Here's how the part is built. I have some questions about the finished solid (model axes, mm). Face numbers are marked on the shaded views. A direction names the side the tool comes from. Give positions to 0.01 mm unless a question says otherwise; leave off trailing zeros. Write each loop counter-clockwise with the first axis right and the second up, starting at its lowest first coordinate (ties: lowest second). Pieces come first, ordered by that corner, then holes. Notation, with made-up numbers: (16.5, 16.5) - (60.5, 16.5) arc R27 cw to (60.5, 52.5) - close; hole circle Ø9 at (29.5, 27.25). An arc over 180 degrees is marked (long way). One line per item, written item: value. Start each with the question number.
1) Imagine slicing it at D-D on z = 35. Write out the boundary of the cut face in (x, y).
2) We'd pull the mould along Y, two halves only. Please class the marked faces 1, 2, 3 and 4: +Y half, -Y half, draft (parallel to the pull), parting line (faces both ways), or undercut.
3) I'm going to push flat-ended pins straight in: P1, Ø7.5, axis at x = 95.25, z = 25.4, coming from the -Y side; P2, Ø10, axis at y = -53.5, z = 12, coming from the +X side; P3, Ø10, axis at x = 77, z = 36.5, coming from the +Y side. Where does each tip first touch, or does it pass through?
4) Imagine slicing it at B-B on y = 8. Write out the boundary of the cut face in (x, z).
5) On a 3-axis mill with a long thin cutter (end or side, diameter ignored), from which of +Z, -Z, +X, -X, +Y, -Y can I reach the whole of each face in a straight line? I mean the marked faces 5, 6, 7, 8 and 9. Say none if no direction works.
6) Imagine slicing it at A-A on z = 25.4. Write out the boundary of the cut face in (x, y).
7) Please list where these lines run through material, in increasing order: L1, parallel to X at y = 28, z = 25; L2, parallel to Z at x = 95.25, y = 29.5; L3, parallel to X at y = 30.5, z = 38.5. Write a range as [from, to].
from build123d import *

# Parameters (mm, degrees)
F0_W     = 127
F0_H     = 127
F0_W_2   = 50.8
F0_H_2   = 6.35
F1_DEPTH = 50.8
F2_R     = 6.35
F3_DEPTH = 101.601


with BuildPart() as f1:
    # F0 (on Top) → F1 (new body)
    with BuildSketch(Plane.XY):
        Polygon((-69.85, -69.85), (69.85, -69.85), (69.85, -31.75), (69.85, -25.4), (69.85, 25.4), (69.85, 31.75), (69.85, 69.85), (-69.85, 69.85), align=None)
        Rectangle(F0_W, F0_H, mode=Mode.SUBTRACT)
        with Locations((95.25, -28.575)):
            Rectangle(F0_W_2, F0_H_2)
        with Locations((95.25, 28.575)):
            Rectangle(F0_W_2, F0_H_2)
    extrude(amount=F1_DEPTH)

    # F2 (on face) → F3 (cut, through all)
    with BuildSketch(Plane.XZ.offset(31.75)):
        with Locations((95.25, 25.4)):
            Circle(F2_R)
    extrude(amount=-F3_DEPTH, mode=Mode.SUBTRACT)


solid = f1.part
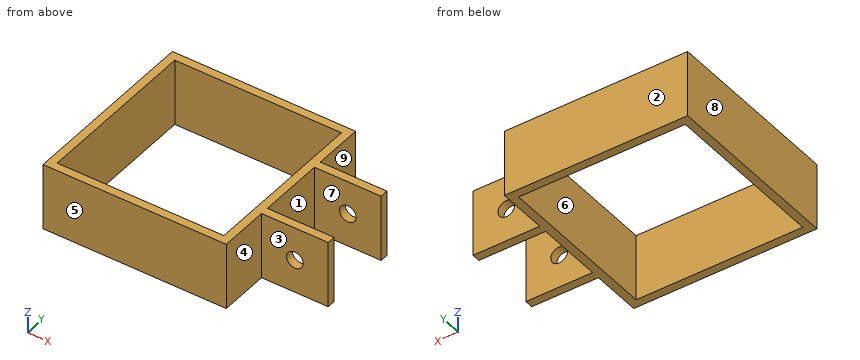
Numbers:
1. outline: (-69.85, -69.85) - (69.85, -69.85) - (69.85, -31.75) - (120.65, -31.75) - (120.65, -25.4) - (69.85, -25.4) - (69.85, 25.4) - (120.65, 25.4) - (120.65, 31.75) - (69.85, 31.75) - (69.85, 69.85) - (-69.85, 69.85) - close; hole (-63.5, -63.5) - (63.5, -63.5) - (63.5, 63.5) - (-63.5, 63.5) - close
2. face 1: undercut
2. face 2: +Y half
2. face 3: -Y half
2. face 4: draft
3. P1: through
3. P2: x = 69.85
3. P3: y = 31.75
4. outline: (-69.85, 0) - (-63.5, 0) - (-63.5, 50.8) - (-69.85, 50.8) - close; (63.5, 0) - (69.85, 0) - (69.85, 50.8) - (63.5, 50.8) - close
5. face 5: +Z, -Z, +X, -X, -Y
5. face 6: +Z, -Z
5. face 7: +Z, -Z, +X
5. face 8: +Z, -Z, -X, +Y, -Y
5. face 9: +Z, -Z, +X, +Y
6. outline: (-69.85, -69.85) - (69.85, -69.85) - (69.85, -31.75) - (88.9, -31.75) - (88.9, -25.4) - (69.85, -25.4) - (69.85, 25.4) - (88.9, 25.4) - (88.9, 31.75) - (69.85, 31.75) - (69.85, 69.85) - (-69.85, 69.85) - close; (101.6, -31.75) - (120.65, -31.75) - (120.65, -25.4) - (101.6, -25.4) - close; (101.6, 25.4) - (120.65, 25.4) - (120.65, 31.75) - (101.6, 31.75) - close; hole (-63.5, -63.5) - (63.5, -63.5) - (63.5, 63.5) - (-63.5, 63.5) - close
7. L1: [-69.85, -63.5], [63.5, 88.91], [101.59, 120.65]
7. L2: [0, 19.05], [31.75, 50.8]
7. L3: [-69.85, -63.5], [63.5, 120.65]
